from build123d import *

# Parameters (mm, degrees)
SKETCH1_W           = 152.4
SKETCH1_H           = 152.4
SKETCH1_W_2         = 20.32
SKETCH1_H_2         = 20.32
SKETCH1_W_3         = 19.05
SKETCH1_H_3         = 19.05
SKETCH1_W_4         = 17.78
SKETCH1_H_4         = 17.78
BOSS_EXTRUDE1_DEPTH = 19.05
SKETCH2_R           = 1.905
SKETCH2_R_2         = 3.175
SKETCH2_R_3         = 4.445
CUT_EXTRUDE1_DEPTH  = 2.54


with BuildPart() as part:
    # Sketch1 → Boss-Extrude1 (new body)
    with BuildSketch(Plane(origin=(0, 0, 0), x_dir=(1, 0, 0), z_dir=(0, 1, 0))):
        Rectangle(SKETCH1_W, SKETCH1_H)
        with Locations((-86.36, -38.1)):
            Rectangle(SKETCH1_W_2, SKETCH1_H_2)
        with Locations((-86.36, 38.1)):
            Rectangle(SKETCH1_W_2, SKETCH1_H_2)
        with Locations((-38.1, 85.725)):
            Rectangle(SKETCH1_W_3, SKETCH1_H_3)
        with Locations((38.1, 85.725)):
            Rectangle(SKETCH1_W_3, SKETCH1_H_3)
        with Locations((85.09, 38.1)):
            Rectangle(SKETCH1_W_4, SKETCH1_H_4)
        with Locations((85.09, -38.1)):
            Rectangle(SKETCH1_W_4, SKETCH1_H_4)
    extrude(amount=BOSS_EXTRUDE1_DEPTH)

    # Sketch2 → Cut-Extrude1 (cut)
    with BuildSketch(Plane(origin=(0, 19.05, 0), x_dir=(1, 0, 0), z_dir=(0, 1, 0))):
        with Locations(Location((63.5, 0, 0), (0, 0, 270))):
            Circle(SKETCH2_R)
        with Locations(Location((0, 63.5, 0), (0, 0, 270))):
            Circle(SKETCH2_R_2)
        with Locations(Location((-63.5, 0, 0), (0, 0, 270))):
            Circle(SKETCH2_R_3)
    extrude(amount=-CUT_EXTRUDE1_DEPTH, mode=Mode.SUBTRACT)


solid = part.part
Check sheet for the modelled part. Datum: model origin and axes. Units: mm. A direction names the side the tool comes from. Round coordinates to 2 decimals unless told otherwise and drop trailing zeros. Write each loop counter-clockwise with the first axis right and the second up, starting at its lowest first coordinate (ties: lowest second). Pieces come first, ordered by that corner, then holes. Notation, with made-up numbers: (-28.5, 64.25) -> (17.5, 64.25) arc R12 ccw to (17.5, 74.25) -> close; hole circle Ø2 at (44.5, 57). An arc over 180 degrees is marked (long way). Answer as CSV lines item,"result". Start each with the question number.
1) Material ranges on line 1 (X direction, y = 17.85, z = 0) (3 decimals); line 2 (Z direction, x = -85, y = 17); line 3 (X direction, y = 17.2, z = -63.5) (3 decimals), recorded low to high. Write a range as from..to.
2) Tool access check on faces 1 (the cylindrical face through (-67.84, 17.8, -0.96)), 2 (the flat face through (-76.2, 9, 0)), 3 (the flat face through (85, 9, 46.99)). Record the directions out of +Z, -Z, +X, -X, +Y, -Y that give a thin tool (end or side, any length) a straight path to the whole face; none if there is none.
3) Section check D-D on x = 0. Enter the section's corners in (y, z) (3 decimals).
4) Release check for a two-part mould opening along Z. For faces 4 (the flat face through (38, 9, -95.25)), 5 (the flat face through (-87, 9, 27.94)), 6 (the flat face through (-47.625, 9, -86)) record: pulls with the +Z half, pulls with the -Z half, needs draft (parallel to the pull), parting line crosses it, or undercut.
5) Go/stop test with flat-tipped pins: P1, Ø1.9, axis at x = 64, z = -0.5, coming from the +Y side; P2, Ø5.5, axis at y = 12, z = -0.5, coming from the -X side; P3, Ø5.5, axis at y = 13.5, z = -11.5, coming from the +X side. Record where each tip stops, or that it passes through.
6) Section check A-A on x = -63.5. Enter the section's corners in (y, z) (3 decimals).
7) Section check C-C on z = -17. Enter the section's corners in (x, y).
8) Section check B-B on y = 9.75. Enter the section's corners in (x, z) (3 decimals), and give its area (3 significant figures).
Found:
1,line 1,"x = -76.2..-67.945, -59.055..61.595, 65.405..76.2"
1,line 2,"z = -48.26..-27.94, 27.94..48.26"
1,line 3,"x = -76.2..-3.175, 3.175..76.2"
2,face 1,"+Y"
2,face 2,"-X, +Y, -Y"
2,face 3,"+Z, +X, +Y, -Y"
3,outline,"(0, -76.2) -> (19.05, -76.2) -> (19.05, -66.675) -> (16.51, -66.675) -> (16.51, -60.325) -> (19.05, -60.325) -> (19.05, 76.2) -> (0, 76.2) -> close"
4,face 4,"pulls with the -Z half"
4,face 5,"undercut"
4,face 6,"needs draft"
5,P1,"stops at y = 16.51"
5,P2,"stops at x = -76.2"
5,P3,"stops at x = 76.2"
6,outline,"(0, -76.2) -> (19.05, -76.2) -> (19.05, -4.445) -> (16.51, -4.445) -> (16.51, 4.445) -> (19.05, 4.445) -> (19.05, 76.2) -> (0, 76.2) -> close"
7,outline,"(-76.2, 0) -> (76.2, 0) -> (76.2, 19.05) -> (-76.2, 19.05) -> close"
8,outline,"(-96.52, -48.26) -> (-76.2, -48.26) -> (-76.2, -76.2) -> (-47.625, -76.2) -> (-47.625, -95.25) -> (-28.575, -95.25) -> (-28.575, -76.2) -> (28.575, -76.2) -> (28.575, -95.25) -> (47.625, -95.25) -> (47.625, -76.2) -> (76.2, -76.2) -> (76.2, -46.99) -> (93.98, -46.99) -> (93.98, -29.21) -> (76.2, -29.21) -> (76.2, 29.21) -> (93.98, 29.21) -> (93.98, 46.99) -> (76.2, 46.99) -> (76.2, 76.2) -> (-76.2, 76.2) -> (-76.2, 48.26) -> (-96.52, 48.26) -> (-96.52, 27.94) -> (-76.2, 27.94) -> (-76.2, -27.94) -> (-96.52, -27.94) -> close"
8,area,"25,400 mm^2"
